```python
from build123d import *

# Parameters (mm, degrees)
F0_W     = 1924.05
F0_H     = 19.05
F1_DEPTH = 241.3
F3_DEPTH = 241.301
F4_W     = 19.05
F4_H     = 12.7
F4_H_2   = 6.35
F5_DEPTH = 241.301


with BuildPart() as f1:
    # F0 (on Front) → F1 (new body)
    with BuildSketch(Plane.XZ):
        Rectangle(F0_W, F0_H)
    extrude(amount=F1_DEPTH)

    # F2 (on face) → F3 (cut, through all)
    with BuildSketch(Plane.XZ.offset(241.3)):
        Polygon((-942.975, -9.525), (-962.025, 9.525), (-962.025, -9.525), align=None)
    extrude(amount=-F3_DEPTH, mode=Mode.SUBTRACT)

    # F4 (on face) → F5 (cut, through all)
    with BuildSketch(Plane.XZ.offset(241.3)):
        with Locations((-571.5, -9.525)):
            Rectangle(F4_W, F4_H)
        with Locations((-190.5, -9.525)):
            Rectangle(F4_W, F4_H)
        with Locations((571.5, -9.525)):
            Rectangle(F4_W, F4_H)
        with Locations((190.5, -9.525)):
            Rectangle(F4_W, F4_H)
        with Locations((952.5, -6.35)):
            Rectangle(F4_W, F4_H_2)
    extrude(amount=-F5_DEPTH, mode=Mode.SUBTRACT)


solid = f1.part
```
Design review of the part built by this model. Coordinates are the model's own, in mm. Give positions to 0.01 mm unless a question says otherwise; leave off trailing zeros. Loops run counter-clockwise (first coordinate to the right, second up) from the corner with the lowest first, then second, coordinate; pieces in that order, holes last. Notation, with made-up numbers: (85, 12.5) -> (118, 12.5) arc R32 ccw to (118, 39.5) -> close; hole circle Ø8 at (84.25, -6.5). An arc over 180 degrees is marked (long way). One line per item, written item: value.
Q1. We need section B-B on z = -6.25. Give the boundary of the cut face in (x, y) (3 decimals).
Numbers:
outline: (-946.25, -241.3) -> (-581.025, -241.3) -> (-581.025, 0) -> (-946.25, 0) -> close; (-561.975, -241.3) -> (-200.025, -241.3) -> (-200.025, 0) -> (-561.975, 0) -> close; (-180.975, -241.3) -> (180.975, -241.3) -> (180.975, 0) -> (-180.975, 0) -> close; (200.025, -241.3) -> (561.975, -241.3) -> (561.975, 0) -> (200.025, 0) -> close; (581.025, -241.3) -> (942.975, -241.3) -> (942.975, 0) -> (581.025, 0) -> close
Q2. For L1, parallel to X at y = -116.5, z = -5.25 (3 decimals); L2, parallel to X at y = -181, z = -4.5 (3 decimals); L3, parallel to Z at x = 185, y = -19 (3 decimals), list the stretches that pass through material, from the lowest coordinate up.
Numbers:
L1: x = -947.25 to -581.025, -561.975 to -200.025, -180.975 to 180.975, 200.025 to 561.975, 581.025 to 942.975
L2: x = -948 to -581.025, -561.975 to -200.025, -180.975 to 180.975, 200.025 to 561.975, 581.025 to 942.975
L3: z = -3.175 to 9.525
Q3. We need section A-A on y = -207. Give the boundary of the cut face in (x, z) (3 decimals), and give its area (3 significant figures).
Numbers:
outline: (-962.025, 9.525) -> (-942.975, -9.525) -> (-581.025, -9.525) -> (-581.025, -3.175) -> (-561.975, -3.175) -> (-561.975, -9.525) -> (-200.025, -9.525) -> (-200.025, -3.175) -> (-180.975, -3.175) -> (-180.975, -9.525) -> (180.975, -9.525) -> (180.975, -3.175) -> (200.025, -3.175) -> (200.025, -9.525) -> (561.975, -9.525) -> (561.975, -3.175) -> (581.025, -3.175) -> (581.025, -9.525) -> (942.975, -9.525) -> (942.975, -3.175) -> (962.025, -3.175) -> (962.025, 9.525) -> close
area: 35,900 mm^2
Q4. For pin 1 Ø1.9 at (y, z) = (-97.5, -7.5) entering from +X (3 decimals); pin 2 Ø3 at (y, z) = (-149.5, -6.5) entering from -X; pin 3 Ø1.5 at (y, z) = (-217, -5) entering from -X, all flat-tipped, find the tip position at first contact; note any pin that passes through.
Numbers:
pin 1: stops at x = 942.975
pin 2: stops at x = -947.5
pin 3: stops at x = -948.25
